The listing builds one solid part. Answer for the finished solid, in the listing's coordinates (mm). Face numbers are marked on the shaded views. A direction names the side the tool comes from. Round coordinates to 2 decimals unless told otherwise and drop trailing zeros. Loops run counter-clockwise (first coordinate to the right, second up) from the corner with the lowest first, then second, coordinate; pieces in that order, holes last. Notation, with made-up numbers: M 86,-25 L 119,-25 A8 cw 119,-18 Z; hole C 38.5,77.25 d10. An arc over 180 degrees is marked long. Answer as a JSON object with one key per item and string values.
Autodesk Inventor part; units mm, degrees
ref_plane "YZ Plane" through (0, 0, 0) normal (1, 0, 0) x (0, 1, 0)
ref_plane "XZ Plane" through (0, 0, 0) normal (0, 1, 0) x (-1, 0, 0)
ref_plane "XY Plane" through (0, 0, 0) normal (0, 0, 1) x (1, 0, 0)
sketch "Sketch1" plane through (0, 0, 0) normal (0, 1, 0) x (-1, 0, 0)
  line L0 (0, 0) -> (0, 16.8)
  line L1 (0, 16.8) -> (-2, 16.8)
  line L2 (-2, 16.8) -> (-2, 10.8)
  line L3 (-2, 10.8) -> (-3, 10.8)
  line L4 (-3, 10.8) -> (-3, 2.8)
  line L5 (-3, 2.8) -> (-5, 2.8)
  line L6 (-5, 2.8) -> (-5, 0)
  line L7 (-5, 0) -> (0, 0)
  dimension "d0" = 10
  dimension "d1" = 6
  dimension "d2" = 4
  dimension "d3" = 6
  dimension "d4" = 8
  dimension "d5" = 2.8
revolve "Revolution1" add sketch "Sketch1" angle 360 about axis through (0, 0, 0) along (0, 0, 1)
thread "Thread1"
sketch "Sketch2" plane through (0, 0, 0) normal (0, 0, -1) x (-1, 0, 0)
  line L0 (0, 1.4434) -> (1.25, 0.7217)
  line L1 (1.25, 0.7217) -> (1.25, -0.7217)
  line L2 (1.25, -0.7217) -> (0, -1.4434)
  line L3 (0, -1.4434) -> (-1.25, -0.7217)
  line L4 (-1.25, -0.7217) -> (-1.25, 0.7217)
  line L5 (-1.25, 0.7217) -> (0, 1.4434)
  point P0 (0, 0)
  point P1 (0, 0)
  dimension "d9" = 2.5
extrude "Extrusion1" cut sketch "Sketch2" against normal blind 2
chamfer "Chamfer1" distance 0.43 angle 45 1 edges at (-2, 0, 16.8)
properties part number "DBSY4-8-6" material "Stainless Steel AISI 304"
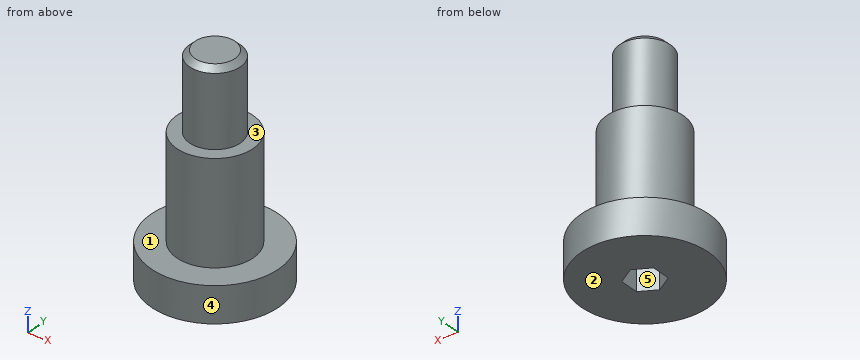
Item 1: The part is cut by section A-A (y = 0). Give the vertices of the cut face in (x, z), then the cut area to 3 significant figures.
Values follow:
{"outline": "M -5,0 L -1.25,0 L -1.25,2 L 1.25,2 L 1.25,0 L 5,0 L 5,2.8 L 3,2.8 L 3,10.8 L 2,10.8 L 2,16.37 L 1.57,16.8 L -1.57,16.8 L -2,16.37 L -2,10.8 L -3,10.8 L -3,2.8 L -5,2.8 Z", "area": "94.8 mm^2"}
Item 2: The part is cut by section B-B (z = 4.25). Give the vertices of the cut face in (x, y), then the cut area to 3 significant figures.
Values follow:
{"outline": "C 0,0 d6", "area": "28.3 mm^2"}
Item 3: Flat-ended cylindrical pins translate along their axes: P1, Ø0.8, axis at x = -0.5, y = 0.5, coming from the -Z side; P2, Ø4, axis at x = -1.5, z = 5.5, coming from the +Y side; P3, Ø6, axis at y = 2, z = 8, coming from the -X side. Find the tip coordinate at first contact, or state that the pin passes through.
Values follow:
{"P1": "z = 2", "P2": "y = 3", "P3": "x = -3"}
Item 4: The part is cut by section C-C (x = -4). Give the vertices of the cut face in (y, z).
Values follow:
{"outline": "M -3,0 L 3,0 L 3,2.8 L -3,2.8 Z"}
Item 5: Which of the six approach directions +Z, -Z, +X, -X, +Y, -Y give full straight-line access (tool end or side, diameter ignored) to the marked faces 1 and 2?
Values follow:
{"face 1": "+Z", "face 2": "-Z, +X, -X, +Y, -Y"}
Item 6: Straight lines are drawn through the part: line 1 (Z direction, x = -3, y = -1.5); line 2 (Z direction, x = 2, y = 0.75); line 3 (X direction, y = -1, z = 1.75). For each, find the intervals that lie inside material, in ascending order.
Values follow:
{"line 1": "0 to 2.8", "line 2": "0 to 10.8", "line 3": "-4.9 to -0.77, 0.77 to 4.9"}
Item 7: Determine the mould class of the marked faces 3, 4 and 5 for opening direction X: released by +X, released by -X, zero draft, split by the parting line, or undercut.
Values follow:
{"face 3": "zero draft", "face 4": "split by the parting line", "face 5": "undercut"}
